Read the model definition and answer for the solid it produces. Units are mm, in the model's axes. Coordinates: 2 decimals unless noted, no trailing zeros. Order: outer loops, then holes, each group sorted by start corner. A loop starts at its lowest first (then second) coordinate and runs counter-clockwise, first axis right, second up. Notation, with made-up numbers: (13.25, 39.5) -> (62.25, 39.5) arc R12 cw to (62.25, 51.5) -> close; hole circle Ø9 at (-35, -19). An arc over 180 degrees is marked (long way). Use CSV: the item, a comma, the result in double quotes.
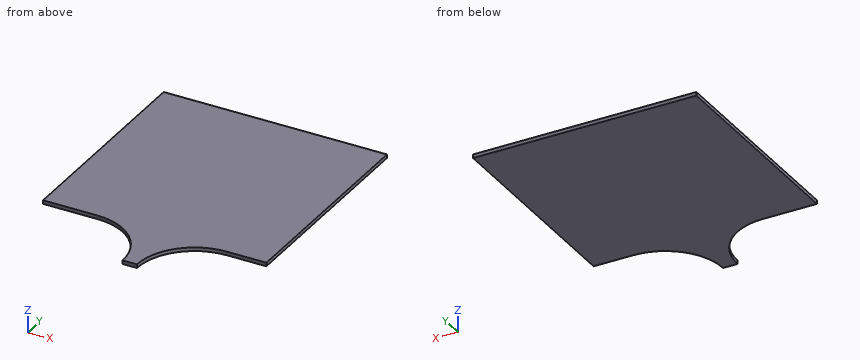
```python
from build123d import *

# Parameters (mm, degrees)
F0_W     = 49.2125
F0_H     = 47.625
F1_DEPTH = 0.79375
F2_W     = 3.175
F2_H     = 12.7
F3_DEPTH = 0.79375
F4_R     = 12.69999


# Not quite as in the source:
# - a fillet or chamfer is up to 0.001 mm smaller than in the source, because OpenCascade refuses the exact size


with BuildPart() as f1:
    # F0 (on Top) → F1 (new body)
    with BuildSketch(Plane.XY):
        with Locations((-36.0471457243, -42.5785098099)):
            Rectangle(F0_W, F0_H)
    extrude(amount=F1_DEPTH)

    # F2 (on face) → F3 (join)
    with BuildSketch(Plane.XY.offset(0.79375)):
        with Locations((-34.4596457243, -72.7410098099)):
            Rectangle(F2_W, F2_H)
    extrude(amount=-F3_DEPTH)

    # F4 (radius 12.7 in the source; OpenCascade refuses exactly that, so slightly less here)
    f4_edges = [f1.edges().sort_by_distance(p)[0] for p in [
        (-36.047146, -66.39101, 0.396875),
        (-32.872146, -66.39101, 0.396875),
    ]]
    fillet(f4_edges, radius=F4_R)


solid = f1.part
```
Item 1: Find section B-B, the plane x = -50.5. Give the vertices of the cut face in (y, z).
Return value:
outline,"(-66.39, 0) -> (-18.77, 0) -> (-18.77, 0.79) -> (-66.39, 0.79) -> close"
Item 2: Find section C-C, the plane y = -75. Give the vertices of the cut face in (x, z).
Return value:
outline,"(-36.72, 0) -> (-32.2, 0) -> (-32.2, 0.79) -> (-36.72, 0.79) -> close"
Item 3: Straight lines are drawn through the part: line 1 along Y through (x, z) = (-22, 0.5); line 2 along Y through (x, z) = (-26, 0.65); line 3 along X through (y, z) = (-74.5, 0.55). For each, find the intervals that lie inside material, in ascending order.
Return value:
line 1,"y = -66.52 to -18.77"
line 2,"y = -67.81 to -18.77"
line 3,"x = -36.91 to -32.01"
Item 4: This flat-tipped pin is pushed along its axis until it touches: P1, Ø12, axis at x = -38, y = -32.5, coming from the -Z side. Where does it stop, or does it pass through?
Return value:
P1,"stops at z = 0"
